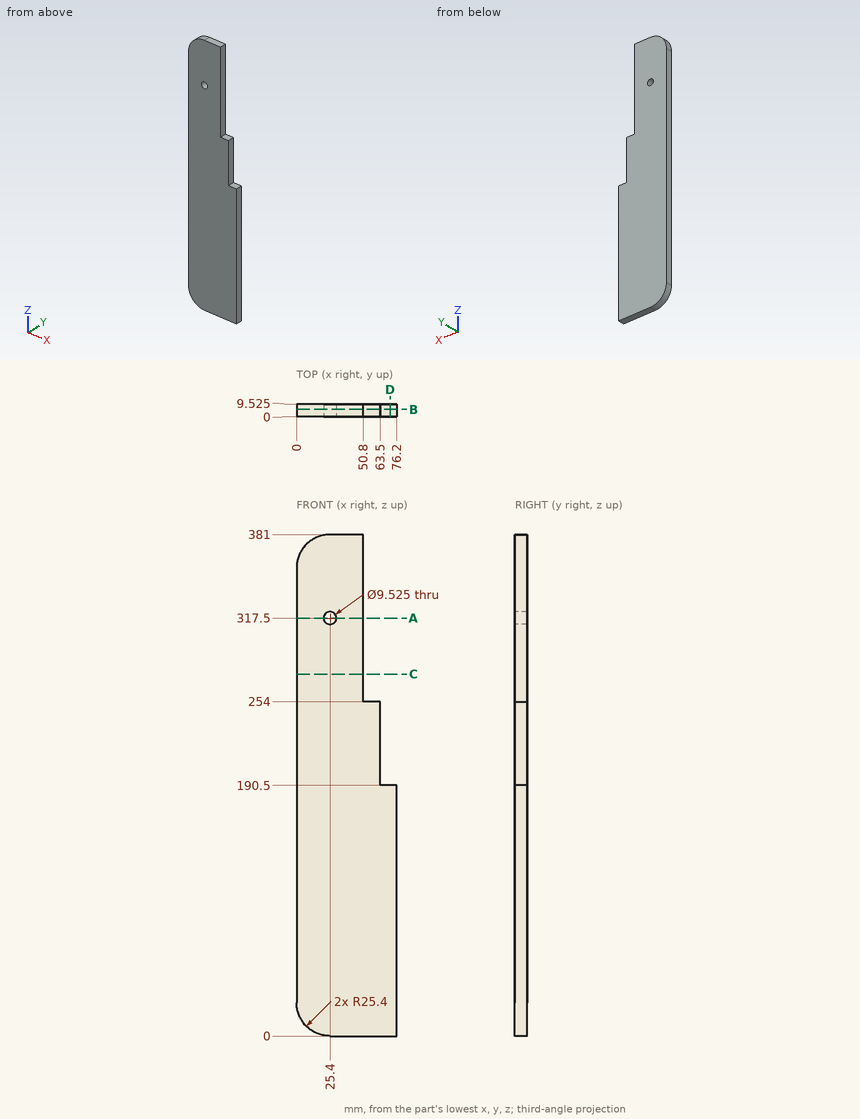
Could you check a few things on this drawing? It's one solid part, dimensions in mm from its lowest x, y, z. Give positions to 0.01 mm unless a question says otherwise; leave off trailing zeros. Order: outer loops, then holes, each group sorted by start corner. A loop starts at its lowest first (then second) coordinate and runs counter-clockwise, first axis right, second up. Notation, with made-up numbers: (60.5, 32) - (81.5, 32) arc R17 ccw to (81.5, 51) - close; hole circle Ø9 at (-37, -13). An arc over 180 degrees is marked (long way). Return JSON: item names as keys, results as strings. Group by question number.
Q1. Suppose I cut it at D-D, the plane x = 71. Please give me the cut outline in (y, z) (3 decimals), and give its area (3 significant figures).
Q2. Suppose I cut it at A-A, the plane z = 317.5. Please give me the cut outline in (x, y) (1 decimal), and give its area (3 significant figures).
Q3. Will these pins go through, and if not, where does the flat tip stop? pin 1 Ø1 at (y, z) = (6, 253.5) entering from +X; pin 2 Ø5 at (x, y) = (15, 2.5) entering from +Z; pin 3 Ø7.5 at (x, z) = (25.4, 317.5) entering from +Y; pin 4 Ø3 at (y, z) = (5, 326.5) entering from +X.
Q4. Please list where these lines run through material, in increasing order: line 1 along X through (y, z) = (2.75, 317.5); line 2 along Z through (x, y) = (25.4, 5.75); line 3 along Z through (x, y) = (61, 8.25). Write a range as [from, to].
Q5. Suppose I cut it at C-C, the plane z = 275. Please give me the cut outline in (x, y) (3 decimals), and give its area (3 significant figures).
Q6. Suppose I cut it at B-B, the plane y = 5.5. Please give me the cut outline in (x, z) (1 decimal), and give its area (3 significant figures).
Resolved:
{
 "1": {"outline": "(0, 0) - (9.525, 0) - (9.525, 190.5) - (0, 190.5) - close", "area": "1,810 mm2"},
 "2": {"outline": "(0, 0) - (20.6, 0) - (20.6, 9.5) - (0, 9.5) - close; (30.2, 0) - (50.8, 0) - (50.8, 9.5) - (30.2, 9.5) - close", "area": "393 mm2"},
 "3": {"pin 1": "stops at x = 63.5", "pin 2": "stops at z = 379.74", "pin 3": "passes through", "pin 4": "stops at x = 50.8"},
 "4": {"line 1": "x = [0, 20.64], [30.16, 50.8]", "line 2": "z = [0, 312.74], [322.26, 381]", "line 3": "z = [0, 254]"},
 "5": {"outline": "(0, 0) - (50.8, 0) - (50.8, 9.525) - (0, 9.525) - close", "area": "484 mm2"},
 "6": {"outline": "(0, 25.4) arc R25.4 ccw to (25.4, 0) - (76.2, 0) - (76.2, 190.5) - (63.5, 190.5) - (63.5, 254) - (50.8, 254) - (50.8, 381) - (25.4, 381) arc R25.4 ccw to (0, 355.6) - close; hole circle Ø9.5 at (25.4, 317.5)", "area": "24,700 mm2"}
}
